Part model, mm, in its own coordinate system. A direction names the side the tool comes from. Round coordinates to 2 decimals unless told otherwise and drop trailing zeros. Loops run counter-clockwise (first coordinate to the right, second up) from the corner with the lowest first, then second, coordinate; pieces in that order, holes last. Notation, with made-up numbers: (-36, 19) -> (-21, 19) arc R28 ccw to (-21, 50) -> close; hole circle Ø5 at (40, -6). An arc over 180 degrees is marked (long way). Answer as a JSON object with one key per item and string values. Group by question number.
from build123d import *

# Parameters (mm, degrees)
SKETCH_1_W                 = 44
SKETCH_1_H                 = 78
EXTRUDE_1_DEPTH            = 57
SHELL_1_T                  = -3
SHELL_1_THICKNESS_2_FACE_W = 75
SHELL_1_THICKNESS_2_FACE_H = 38
SHELL_1_THICKNESS_2_DEPTH  = 7
SKETCH_3_R                 = 3.6
CUT_EXTRUDE_1_DEPTH        = 4.1
CUT_EXTRUDE_2_REACH        = 66.915
SKETCH_4_R                 = 2.25
SKETCH_5_W                 = 3
SKETCH_5_H                 = 3
CUT_EXTRUDE_3_DEPTH        = 6
SKETCH_6_W                 = 8
SKETCH_6_H                 = 8
SKETCH_6_R                 = 1.75
EXTRUDE_2_DEPTH            = 8
CUT_EXTRUDE_4_DEPTH        = 2.6
CUT_EXTRUDE_5_REACH        = 100.864
SKETCH_8_R                 = 5


with BuildPart() as part:
    # 草圖1 → 填料-伸長1 (new body)
    with BuildSketch(Plane(origin=(0, 0, 0), x_dir=(1, 0, 0), z_dir=(0, 1, 0))):
        Rectangle(SKETCH_1_W, SKETCH_1_H)
    extrude(amount=EXTRUDE_1_DEPTH)

    # 薄殼1
    shell_1_openings = [part.faces().sort_by_distance(p)[0] for p in [
        (0, 28.5, 39),
    ]]
    offset(amount=SHELL_1_T, openings=shell_1_openings, kind=Kind.INTERSECTION)

    # 薄殼1 thickness 2 face (on inner face of the shell) → 薄殼1 thickness 2 (add)
    with BuildSketch(Plane(origin=(0, 3, 1.5), x_dir=(0, 0, -1), z_dir=(0, -1, 0))):
        Rectangle(SHELL_1_THICKNESS_2_FACE_W, SHELL_1_THICKNESS_2_FACE_H)
    extrude(amount=-SHELL_1_THICKNESS_2_DEPTH)

    # 草圖3 → 除料-伸長1 (cut)
    with BuildSketch(Plane(origin=(0, 10, 0), x_dir=(1, 0, 0), z_dir=(0, 1, 0))):
        with Locations(Location((0, 25, 0), (0, 0, 270))):
            Circle(SKETCH_3_R)
        with Locations(Location((0, -29, 0), (0, 0, 270))):
            Circle(SKETCH_3_R)
    extrude(amount=-CUT_EXTRUDE_1_DEPTH, mode=Mode.SUBTRACT)

    # 草圖4 → 除料-伸長2 (cut, up to next)
    with BuildSketch(Plane(origin=(0, 10, 0), x_dir=(1, 0, 0), z_dir=(0, 1, 0)), mode=Mode.PRIVATE) as cut_extrude_2_sk1:
        with Locations(Location((0, 25, 0), (0, 0, 270))):
            Circle(SKETCH_4_R)
    cut_extrude_2_tool1 = extrude(cut_extrude_2_sk1.sketch, amount=-CUT_EXTRUDE_2_REACH, mode=Mode.PRIVATE) & part.part
    # 草圖4 → 除料-伸長2 (cut, up to next)
    with BuildSketch(Plane(origin=(0, 10, 0), x_dir=(1, 0, 0), z_dir=(0, 1, 0)), mode=Mode.PRIVATE) as cut_extrude_2_sk2:
        with Locations(Location((0, -29, 0), (0, 0, 270))):
            Circle(SKETCH_4_R)
    cut_extrude_2_tool2 = extrude(cut_extrude_2_sk2.sketch, amount=-CUT_EXTRUDE_2_REACH, mode=Mode.PRIVATE) & part.part
    add(cut_extrude_2_tool1.solids().sort_by_distance((0, 10, -25))[0], mode=Mode.SUBTRACT)
    add(cut_extrude_2_tool2.solids().sort_by_distance((0, 10, 29))[0], mode=Mode.SUBTRACT)

    # 草圖5 → 除料-伸長3 (cut)
    with BuildSketch(Plane.XY.offset(39)):
        with Locations((20.5, 11.5)):
            Rectangle(SKETCH_5_W, SKETCH_5_H)
    extrude(amount=-CUT_EXTRUDE_3_DEPTH, mode=Mode.SUBTRACT)

    # 草圖6 → 填料-伸長2 (add)
    with BuildSketch(Plane.XY.offset(39)):
        with Locations((-26, 53)):
            Rectangle(SKETCH_6_W, SKETCH_6_H)
        with Locations((-26, 53)):
            Circle(SKETCH_6_R, mode=Mode.SUBTRACT)
        with Locations((-26, 4)):
            Rectangle(SKETCH_6_W, SKETCH_6_H)
        with Locations((-26, 4)):
            Circle(SKETCH_6_R, mode=Mode.SUBTRACT)
        with Locations((26, 4)):
            Rectangle(SKETCH_6_W, SKETCH_6_H)
        with Locations(Location((26, 4, 0), (0, 0, 180))):
            Circle(SKETCH_6_R, mode=Mode.SUBTRACT)
        with Locations((26, 53)):
            Rectangle(SKETCH_6_W, SKETCH_6_H)
        with Locations(Location((26, 53, 0), (0, 0, 180))):
            Circle(SKETCH_6_R, mode=Mode.SUBTRACT)
    extrude(amount=-EXTRUDE_2_DEPTH)

    # 草圖7 → 除料-伸長4 (cut)
    with BuildSketch(Plane(origin=(0, 0, 31), x_dir=(-1, 0, 0), z_dir=(0, 0, -1))):
        Polygon((-22.824573519, 53), (-24.41228676, 55.75), (-27.58771324, 55.75), (-29.175426481, 53), (-27.58771324, 50.25), (-24.41228676, 50.25), align=None)
        Polygon((-22.824573519, 4), (-24.41228676, 6.75), (-27.58771324, 6.75), (-29.175426481, 4), (-27.58771324, 1.25), (-24.41228676, 1.25), align=None)
        Polygon((24.41228676, 1.25), (22.824573519, 4), (24.41228676, 6.75), (27.58771324, 6.75), (29.175426481, 4), (27.58771324, 1.25), align=None)
        Polygon((24.41228676, 50.25), (22.824573519, 53), (24.41228676, 55.75), (27.58771324, 55.75), (29.175426481, 53), (27.58771324, 50.25), align=None)
    extrude(amount=-CUT_EXTRUDE_4_DEPTH, mode=Mode.SUBTRACT)

    # 草圖8 → 除料-伸長5 (cut, up to next)
    with BuildSketch(Plane.XY.offset(-36), mode=Mode.PRIVATE) as cut_extrude_5_sk1:
        with Locations((0, 30)):
            Circle(SKETCH_8_R)
    cut_extrude_5_tool1 = extrude(cut_extrude_5_sk1.sketch, amount=-CUT_EXTRUDE_5_REACH, mode=Mode.PRIVATE) & part.part
    add(cut_extrude_5_tool1.solids().sort_by_distance((0, 30, -36))[0], mode=Mode.SUBTRACT)


solid = part.part
Item 1: Drill centre lines: line 1 (Y direction, x = -26, z = 35.4); line 2 (Y direction, x = 4, z = -3); line 3 (X direction, y = 8.4, z = 29). Where is each one in solid material? Low to high.
Item 2: Two-plate mould, pull along Z, no slides. Class faces 4 (the face through (24.6, 5.3, 33.6)), 5 (the face through (0.158, 7.979, -28.597)), 6 (the face through (-26, 55.75, 32)): pulls with the +Z half, pulls with the -Z half, needs draft (parallel to the pull), parting line crosses it, or undercut.
Item 3: Band-saw the part on A-A, the plane x = 0. List the corners of the cut face in (y, z).
Item 4: Drop flat-ended pins along their axis: pin 1 Ø1 at (y, z) = (7, 11) entering from +X; pin 2 Ø13 at (y, z) = (42.5, -6.5) entering from -X; pin 3 Ø1.6 at (x, y) = (-25, 3) entering from -Z. Give the stop position or say it passes through.
Item 5: Which spindle directions (+Z, -Z, +X, -X, +Y, -Y) get a long thin tool onto all of the face, cutting with end or side? Do faces 1 (the face through (2, 5.9, -23)), 2 (the face through (26, 8, 35)), 3 (the face through (19, 32, 2)). Say none if no direction does.
Item 6: Band-saw the part on D-D, the plane x = -26. List the corners of the cut face in (y, z), plus the area to 3 significant figures.
Item 7: Band-saw the part on B-B, the plane z = -31. List the corners of the cut face in (x, y).
Item 8: Band-saw the part on C-C, the plane y = 18. List the corners of the cut face in (x, z).
Entries:
{
 "1": {"line 1": "0 to 2.25, 5.75 to 8, 49 to 51.25, 54.75 to 57", "line 2": "0 to 10, 54 to 57", "line 3": "-22 to -3.6, 3.6 to 22"},
 "2": {"face 4": "pulls with the -Z half", "face 5": "undercut", "face 6": "needs draft"},
 "3": {"outline": "(0, -39) -> (25, -39) -> (25, -36) -> (10, -36) -> (10, -28.6) -> (5.9, -28.6) -> (5.9, -27.25) -> (0, -27.25) -> close; (0, -22.75) -> (5.9, -22.75) -> (5.9, -21.4) -> (10, -21.4) -> (10, 25.4) -> (5.9, 25.4) -> (5.9, 26.75) -> (0, 26.75) -> close; (0, 31.25) -> (5.9, 31.25) -> (5.9, 32.6) -> (10, 32.6) -> (10, 39) -> (0, 39) -> close; (35, -39) -> (57, -39) -> (57, 39) -> (54, 39) -> (54, -36) -> (35, -36) -> close"},
 "4": {"pin 1": "x = 22", "pin 2": "x = -22", "pin 3": "z = 33.6"},
 "5": {"face 1": "none", "face 2": "+Z, -Z, +X", "face 3": "+Z"},
 "6": {"outline": "(0, 31) -> (1.25, 31) -> (1.25, 33.6) -> (2.25, 33.6) -> (2.25, 39) -> (0, 39) -> close; (5.75, 33.6) -> (6.75, 33.6) -> (6.75, 31) -> (8, 31) -> (8, 39) -> (5.75, 39) -> close; (49, 31) -> (50.25, 31) -> (50.25, 33.6) -> (51.25, 33.6) -> (51.25, 39) -> (49, 39) -> close; (54.75, 33.6) -> (55.75, 33.6) -> (55.75, 31) -> (57, 31) -> (57, 39) -> (54.75, 39) -> close", "area": "61.6 mm²"},
 "7": {"outline": "(-22, 0) -> (22, 0) -> (22, 57) -> (-22, 57) -> close; hole (-19, 10) -> (19, 10) -> (19, 54) -> (-19, 54) -> close"},
 "8": {"outline": "(-22, -39) -> (22, -39) -> (22, 39) -> (19, 39) -> (19, -36) -> (-19, -36) -> (-19, 39) -> (-22, 39) -> close"}
}
